from build123d import *

# Parameters (mm, degrees)
CROQUIS2_R              = 0.75
SALIENTE_EXTRUIR1_DEPTH = 2
CROQUIS6_R              = 1.475
SALIENTE_EXTRUIR3_DEPTH = 2
SALIENTE_EXTRUIR4_REACH = 10.975
CROQUIS8_W              = 6
CROQUIS8_H              = 2


with BuildPart() as part:
    # Croquis2 → Saliente-Extruir1 (new body)
    with BuildSketch(Plane(origin=(0, 0, 0), x_dir=(1, 0, 0), z_dir=(0, 1, 0))):
        with BuildLine():
            Line((-2.585, 3), (2.585, 3))
            ThreePointArc((2.585, 3), (3.645660172, 2.560660172), (4.085, 1.5))
            Line((4.085, 1.5), (4.085, -1.5))
            ThreePointArc((4.085, -1.5), (3.645660172, -2.560660172), (2.585, -3))
            Line((2.585, -3), (-2.585, -3))
            Line((-2.585, -3), (-2.585, 3))
        make_face()
        with Locations(Location((-0.915, 0, 0), (0, 0, 270))):
            Circle(CROQUIS2_R, mode=Mode.SUBTRACT)
        with Locations(Location((2.085, 0, 0), (0, 0, 270))):
            Circle(CROQUIS2_R, mode=Mode.SUBTRACT)
    extrude(amount=SALIENTE_EXTRUIR1_DEPTH)



with BuildPart() as body_2:
    # Croquis6 → Saliente-Extruir3 (new body)
    with BuildSketch(Plane(origin=(-0.2925, -0.2925, 0), x_dir=(0, 0, 1), z_dir=(0.7071067811865438, 0.7071067811865512, 0))):
        with BuildLine():
            Line((-3, -3.242084592), (3, -3.242084592))
            Line((3, -3.242084592), (3, -7.582084592))
            ThreePointArc((3, -7.582084592), (0, -10.582084592), (-3, -7.582084592))
            Line((-3, -7.582084592), (-3, -3.242084592))
        make_face()
        with Locations(Location((0, -7.582084592, 0), (0, 0, 270))):
            Circle(CROQUIS6_R, mode=Mode.SUBTRACT)
    extrude(amount=-SALIENTE_EXTRUIR3_DEPTH)


with BuildPart() as part_1:
    add(part.part)

    add(body_2.part)  # Saliente-Extruir4 merges body 2
    # Saliente-Extruir4: up to this plane
    saliente_extruir4_end = Plane(origin=(2.585, 0, 1.5), z_dir=(0, -1, 0))
    # Croquis8 → Saliente-Extruir4 (add, up to the surface)
    with BuildSketch(Plane(origin=(-2.2925, 2.2925, 0), x_dir=(0, 0, -1), z_dir=(0.7071067811865513, -0.7071067811865438, 0)), mode=Mode.PRIVATE) as saliente_extruir4_sk1:
        with Locations((0, -1.413657467)):
            Rectangle(CROQUIS8_W, CROQUIS8_H)
    saliente_extruir4_tool1 = split(extrude(saliente_extruir4_sk1.sketch, amount=SALIENTE_EXTRUIR4_REACH, mode=Mode.PRIVATE), bisect_by=saliente_extruir4_end, keep=Keep.BOTH, mode=Mode.PRIVATE)
    add(saliente_extruir4_tool1.solids().sort_by_distance((-3.292107, 1.292893, 0))[0])


solid = part_1.part
Input: part model. Units: mm. Frame: model coordinates. A direction names the side the tool comes from. Coordinates: 2 decimals unless noted, no trailing zeros. Order: outer loops, then holes, each group sorted by start corner. A loop starts at its lowest first (then second) coordinate and runs counter-clockwise, first axis right, second up. Notation, with made-up numbers: M 14,18.25 L 36,18.25 A4 ccw 36,23.25 Z; hole C 79.25,77.25 d4. An arc over 180 degrees is marked long. Answer in a Markdown table with one row per item.
(1) Section query B-B, the plane z = 1.2. Output: boundary loops of the cut face in (x, y) (3 decimals).
Numbers:
| item | result |
|---|---|
| outline | M -9.012,5.599 L -7.675,4.261 L -6.26,5.675 L -7.598,7.013 Z; M -6.462,3.048 L -3.413,0 L 4.085,0 L 4.085,2 L -2.585,2 L -5.047,4.462 Z |
(2) Draft query along Z for faces 4 (the cylindrical face through (3.634, 0.986, -2.572)), 5 (the flat face through (-1.013, 0.428, 0.01)), 6 (the flat face through (-4.567, 3.982, -0.625)), 7 (the cylindrical face through (-8.472, 6.492, 0.066)). Return one class per face: pulls with the +Z half, pulls with the -Z half, needs draft (parallel to the pull), parting line crosses it, or undercut.
Numbers:
| item | result |
|---|---|
| face 4 | pulls with the -Z half |
| face 5 | undercut |
| face 6 | needs draft |
| face 7 | parting line crosses it |
(3) Contact query for flat-ended pins moving along their axis: pin 1 Ø3 at (y, z) = (4, -0.5) entering from -X; pin 2 Ø1.8 at (x, z) = (2, -0.5) entering from +Y. Output: stop coordinate, or through.
Numbers:
| item | result |
|---|---|
| pin 1 | stops at x = -8.91 |
| pin 2 | stops at y = 2 |
(4) Section query D-D, the plane z = 2.3. Output: boundary loops of the cut face in (x, y) (3 decimals), plus the area to 3 significant figures.
Numbers:
| item | result |
|---|---|
| outline | M -8.43,5.017 L -3.413,0 L 3.854,0 L 3.854,2 L -2.585,2 L -7.016,6.431 Z |
| area | 27.1 mm^2 |
(5) Access query for faces 1 (the flat face through (1, 2, 0)), 2 (the flat face through (-5.7, 2.287, 0.042)), 3 (the cylindrical face through (-0.17, 1.21, -0.1)). Directions: +Z, -Z, +X, -X, +Y, -Y. A direction counts if a zero-diameter tool reaches every point of the face in a straight line with its end or side. Return the directions, or none.
Numbers:
| item | result |
|---|---|
| face 1 | +Z, -Z, +X, +Y |
| face 2 | +Z, -Z, -X, -Y |
| face 3 | +Y |
(6) Section query A-A, the plane z = 0. Output: boundary loops of the cut face in (x, y) (3 decimals).
Numbers:
| item | result |
|---|---|
| outline | M -9.189,5.776 L -8.111,4.698 L -6.697,6.112 L -7.775,7.19 Z; M -6.025,2.612 L -3.413,0 L -0.585,0 L -1.665,1.08 L -1.665,2 L -2.585,2 L -4.611,4.026 Z; M -0.165,0 L 1.335,0 L 1.335,2 L -0.165,2 Z; M 2.835,0 L 4.085,0 L 4.085,2 L 2.835,2 Z |
(7) Material intervals for line 1 (X direction, y = 0.65, z = 0) (3 decimals); line 2 (Y direction, x = -1.75, z = -2.3); line 3 (X direction, y = 0.7, z = 0) (3 decimals), sorted ascending. Write a range as [from, to].
Numbers:
| item | result |
|---|---|
| line 1 | x = [-4.063, -1.235], [-0.165, 1.335], [2.835, 4.085] |
| line 2 | y = [0, 2] |
| line 3 | x = [-4.113, -1.285], [-0.165, 1.335], [2.835, 4.085] |
(8) Section query C-C, the plane x = 0. Output: boundary loops of the cut face in (y, z), plus the area to 3 significant figures.
Numbers:
| item | result |
|---|---|
| outline | M 0,-3 L 2,-3 L 2,3 L 0,3 Z |
| area | 12.0 mm^2 |
